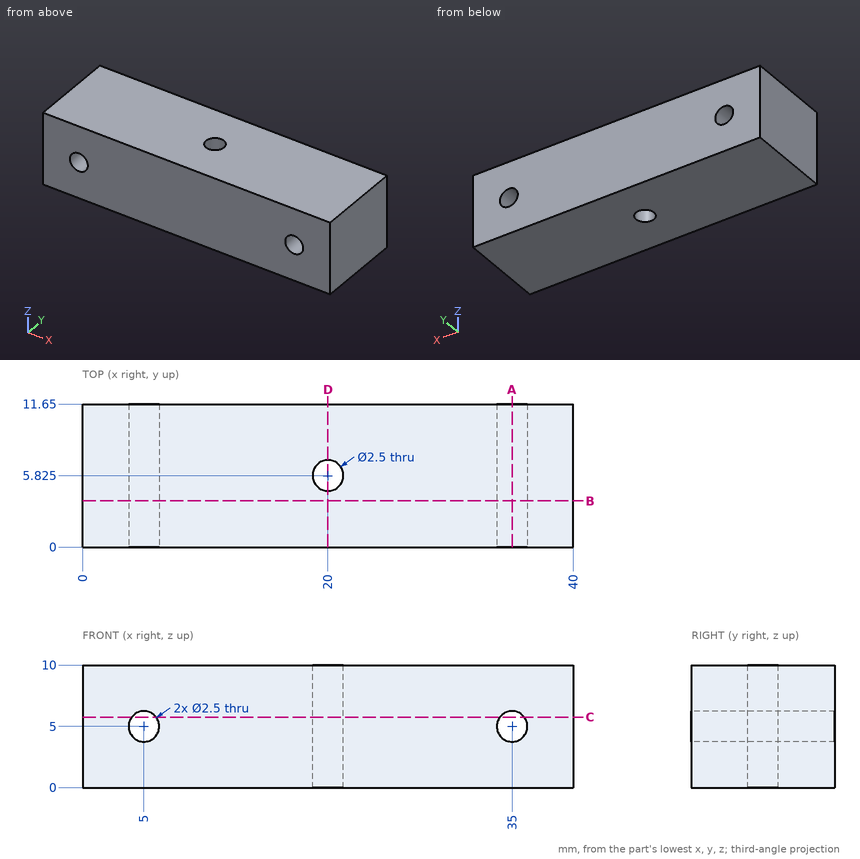
Source: three-view drawing plus pictorial views. Frame: mm from the lowest corner of the part. Coordinates: 2 decimals unless noted, no trailing zeros. Loops run counter-clockwise (first coordinate to the right, second up) from the corner with the lowest first, then second, coordinate; pieces in that order, holes last. Notation, with made-up numbers: (-17, -19.75) -> (-1, -19.75) arc R35 cw to (-1, 13.25) -> close; hole circle Ø5 at (58, -23.5). An arc over 180 degrees is marked (long way). Answer in a Markdown table with one row per item. Add a question column.
Q1. Contact query for flat-ended pins moving along their axis: pin 1 Ø4 at (x, y) = (20, 5.825) entering from +Z; pin 2 Ø2 at (x, z) = (5, 5) entering from +Y. Output: stop coordinate, or through.
Q2. Section B-B on y = 3.75. Return the cut outline in (x, z), and give its area (3 significant figures).
Q3. Section D-D on x = 20. Return the cut outline in (y, z) (3 decimals), and give its area (3 significant figures).
Q4. Ray query, line 1 along X through (y, z) = (2.75, 5); line 2 along Y through (x, z) = (20, 6.5) (3 decimals); line 3 along X through (y, z) = (1, 4.5). Return the intervals inside material, ascending.
Q5. Section A-A on x = 35. Return the cut outline in (y, z), and give its area (3 significant figures).
Q6. Section C-C on z = 5.75. Return the cut outline in (x, y) (3 decimals), and give its area (3 significant figures).
Computed values:
| question | item | result |
|---|---|---|
| 1 | pin 1 | stops at z = 10 |
| 1 | pin 2 | passes through |
| 2 | outline | (0, 0) -> (40, 0) -> (40, 10) -> (0, 10) -> close; hole circle Ø2.5 at (5, 5); hole circle Ø2.5 at (35, 5) |
| 2 | area | 390 mm^2 |
| 3 | outline | (0, 0) -> (4.575, 0) -> (4.575, 10) -> (0, 10) -> close; (7.075, 0) -> (11.65, 0) -> (11.65, 10) -> (7.075, 10) -> close |
| 3 | area | 91.5 mm^2 |
| 4 | line 1 | x = 0 to 3.75, 6.25 to 33.75, 36.25 to 40 |
| 4 | line 2 | y = 0 to 4.575, 7.075 to 11.65 |
| 4 | line 3 | x = 0 to 3.85, 6.15 to 33.85, 36.15 to 40 |
| 5 | outline | (0, 0) -> (11.65, 0) -> (11.65, 3.75) -> (0, 3.75) -> close; (0, 6.25) -> (11.65, 6.25) -> (11.65, 10) -> (0, 10) -> close |
| 5 | area | 87.4 mm^2 |
| 6 | outline | (0, 0) -> (4, 0) -> (4, 11.65) -> (0, 11.65) -> close; (6, 0) -> (34, 0) -> (34, 11.65) -> (6, 11.65) -> close; (36, 0) -> (40, 0) -> (40, 11.65) -> (36, 11.65) -> close; hole circle Ø2.5 at (20, 5.825) |
| 6 | area | 414 mm^2 |
